Verification items for the finished model (mm, model axes). Face numbers are marked on the shaded views. A direction names the side the tool comes from. Coordinates: 2 decimals unless noted, no trailing zeros. Order: outer loops, then holes, each group sorted by start corner. A loop starts at its lowest first (then second) coordinate and runs counter-clockwise, first axis right, second up. Notation, with made-up numbers: (-14.75, -35.5) -> (39.25, -35.5) arc R21 ccw to (39.25, -29.5) -> close; hole circle Ø8 at (-22.5, 56.25). An arc over 180 degrees is marked (long way). Use CSV: the item, a comma, the result in double quotes. Start each with the question number.
1) Release check for a two-part mould opening along Y. For the marked faces 1, 2, 3 and 4 record: released by +Y, released by -Y, zero draft, split by the parting line, or undercut.
2) Sectioned sample at D-D on z = 28. Record the boundary of the cut face in (x, y).
3) Sectioned sample at A-A on x = 0. Give the number of separate pieces and of enclosed holes in the cut face, then the cut area to 3 significant figures.
4) Sectioned sample at B-B on y = 16. Record the boundary of the cut face in (x, z).
5) Sectioned sample at C-C on x = 18.5. Record the boundary of the cut face in (y, z).
6) Go/stop test with flat-tipped pins: pin 1 (2.5 mm diameter, centred on x = 0, y = 12, fed in from +Z); pin 2 (4 mm diameter, centred on x = -3, y = -16.5, fed in from +Z); pin 3 (12 mm diameter, centred on x = 11.5, z = 36, fed in from +Y). Record where each tip stops, or that it passes through.
7) Scan lines: line 1 along Y through (x, z) = (0, 0.25); line 2 along Z through (x, y) = (-4, 18); line 3 along X through (y, z) = (6, 0.75). Record each from-to range of solid material in increasing order.
8) Tool access check on the marked faces 5, 6 and 7. Record the directions out of +Z, -Z, +X, -X, +Y, -Y that give a thin tool (end or side, any length) a straight path to the whole face; none if there is none.
from build123d import *

# Parameters (mm, degrees)
SKETCH_1_R            = 9.25
EXTRUDE_1_DEPTH       = 89.5
SKETCH_4_R            = 12.25
EXTRUDE_2_DEPTH       = 16
SKETCH_5_R            = 21
EXTRUDE_3_DEPTH       = 5
EXTRUDE_4_DEPTH       = 4.2
EXTRUDE_4_DEPTH_BACK  = 4
SKETCH_6_R            = 21
SKETCH_6_R_2          = 2.25
SKETCH_7_R            = 20
CUT_EXTRUDE_1_DEPTH   = 2
SKETCH_8_OUTSIDE_W    = 66.188
SKETCH_8_OUTSIDE_H    = 66.188
CUT_EXTRUDE_4_DEPTH   = 14.5
SKETCH_11_R           = 9.5
EXTRUDE_5_DEPTH       = 50
SKETCH_13_W           = 10
SKETCH_13_H           = 10.246950766
CUT_EXTRUDE_1_2_DEPTH = 50
CHAMFER_1_SIZE        = 0.5


with BuildPart() as part:
    # 草图1 → 凸台-拉伸1 (new body)
    with BuildSketch(Plane.XY):
        with Locations(Location((0, 0, 0), (0, 0, 180))):
            Circle(SKETCH_1_R)
    extrude(amount=EXTRUDE_1_DEPTH)

    # 草图4 → 凸台-拉伸2 (add)
    with BuildSketch(Plane.XY.offset(39.5)):
        Circle(SKETCH_4_R)
    extrude(amount=-EXTRUDE_2_DEPTH)

    # 草图5 → 凸台-拉伸3 (add)
    with BuildSketch(Plane(origin=(0, 0, 23.5), x_dir=(-1, 0, 0), z_dir=(0, 0, -1))):
        Circle(SKETCH_5_R)
    extrude(amount=EXTRUDE_3_DEPTH)

    # 草图6 → 凸台-拉伸4 (add, two sides: drawn at the far end of the back side and taken through both)
    with BuildSketch(Plane(origin=(0, 0, 0), x_dir=(-1, 0, 0), z_dir=(0, 0, -1)).offset(-EXTRUDE_4_DEPTH_BACK)):
        Circle(SKETCH_6_R)
        with Locations((0, 12)):
            Circle(SKETCH_6_R_2, mode=Mode.SUBTRACT)
        with Locations((10.392304845, 6)):
            Circle(SKETCH_6_R_2, mode=Mode.SUBTRACT)
        with Locations((10.392304845, -6)):
            Circle(SKETCH_6_R_2, mode=Mode.SUBTRACT)
        with Locations((0, -12)):
            Circle(SKETCH_6_R_2, mode=Mode.SUBTRACT)
        with Locations((-10.392304845, -6)):
            Circle(SKETCH_6_R_2, mode=Mode.SUBTRACT)
        with Locations((-10.392304845, 6)):
            Circle(SKETCH_6_R_2, mode=Mode.SUBTRACT)
    extrude(amount=EXTRUDE_4_DEPTH + EXTRUDE_4_DEPTH_BACK)

    # 草图7 → Cut-Extrude 1 (cut)
    with BuildSketch(Plane(origin=(0, 0, -4.2), x_dir=(-1, 0, 0), z_dir=(0, 0, -1))):
        Circle(SKETCH_7_R)
    extrude(amount=-CUT_EXTRUDE_1_DEPTH, mode=Mode.SUBTRACT)

    # 草图8 outside → 切除-拉伸4 (cut)
    with BuildSketch(Plane(origin=(0, 0, 18.5), x_dir=(-1, 0, 0), z_dir=(0, 0, -1))):
        Rectangle(SKETCH_8_OUTSIDE_W, SKETCH_8_OUTSIDE_H)
        Polygon((-9.25, 0), (-4.625, -8.010734985), (4.625, -8.010734985), (9.25, 0), (4.625, 8.010734985), (-4.625, 8.010734985), align=None, mode=Mode.SUBTRACT)
    extrude(amount=CUT_EXTRUDE_4_DEPTH, mode=Mode.SUBTRACT)

    # 草图11 → 凸台-拉伸5 (add)
    with BuildSketch(Plane.XY.offset(39.5)):
        Circle(SKETCH_11_R)
    extrude(amount=EXTRUDE_5_DEPTH)

    # 草图13 → Cut-Extrude 1 2 (cut)
    with BuildSketch(Plane.XY.offset(89.5)):
        with Locations((-13, 0)):
            Rectangle(SKETCH_13_W, SKETCH_13_H)
        with Locations((13, 0)):
            Rectangle(SKETCH_13_W, SKETCH_13_H)
    extrude(amount=-CUT_EXTRUDE_1_2_DEPTH, mode=Mode.SUBTRACT)

    # 倒角1
    chamfer_1_edges = [part.edges().sort_by_distance(p)[0] for p in [
        (8, 0, 89.5),
        (0, -9.5, 89.5),
        (-8, 0, 89.5),
        (0, 9.5, 89.5),
    ]]
    chamfer(chamfer_1_edges, length=CHAMFER_1_SIZE)


solid = part.part
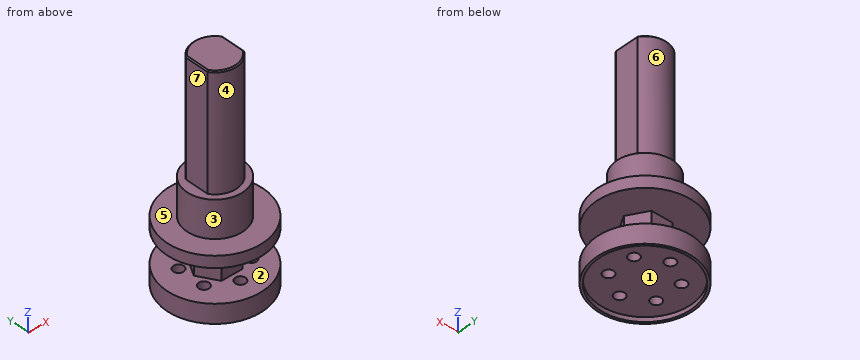
Answers follow:
1,face 1,"undercut"
1,face 2,"zero draft"
1,face 3,"split by the parting line"
1,face 4,"released by -Y"
2,outline,"circle Ø24.5 at (0, 0)"
3,separate pieces,"3"
3,enclosed holes,"0"
3,area,"1,990 mm²"
4,outline,"(-13.6, -4.2) -> (-12, -4.2) -> (-12, -2.2) -> (12, -2.2) -> (12, -4.2) -> (13.6, -4.2) -> (13.6, 4) -> (-13.6, 4) -> close; (-13.6, 18.5) -> (13.6, 18.5) -> (13.6, 23.5) -> (-13.6, 23.5) -> close"
5,outline,"(-9.94, -4.2) -> (-7.6, -4.2) -> (-7.6, -2.2) -> (7.6, -2.2) -> (7.6, -4.2) -> (9.94, -4.2) -> (9.94, 4) -> (-9.94, 4) -> close; (-9.94, 18.5) -> (9.94, 18.5) -> (9.94, 23.5) -> (-9.94, 23.5) -> close"
6,pin 1,"stops at z = 39.5"
6,pin 2,"stops at z = 23.5"
6,pin 3,"stops at y = 10.95"
7,line 1,"y = -21 to -14.25, -9.75 to 9.75, 14.25 to 21"
7,line 2,"z = -2.2 to 4, 18.5 to 23.5"
7,line 3,"x = -20.12 to -12.64, -8.14 to 8.14, 12.64 to 20.12"
8,face 5,"+Z"
8,face 6,"+Z, +Y"
8,face 7,"+Z, -X, +Y, -Y"
